Verification items for the finished model (mm, model axes). Face numbers are marked on the shaded views. A direction names the side the tool comes from. Give positions to 0.01 mm unless a question says otherwise; leave off trailing zeros. Loops run counter-clockwise (first coordinate to the right, second up) from the corner with the lowest first, then second, coordinate; pieces in that order, holes last. Notation, with made-up numbers: M -4.5,52.25 L 11.5,52.25 A26 cw 11.5,76.25 Z; hole C 69,-28.5 d10. An arc over 180 degrees is marked long. Use CSV: the item, a comma, the result in double quotes.
from build123d import *
from build123d.topology import SkipClean

# Parameters (mm, degrees)
BOSS_EXTRUDE1_DEPTH = 35
SKETCH2_W           = 14
SKETCH2_H           = 21
CUT_EXTRUDE1_DEPTH  = 35
BOSS_EXTRUDE2_DEPTH = 35
CUT_EXTRUDE2_DEPTH  = 58
FILLET1_R           = 5
CHAMFER2_SIZE       = 0.5
CHAMFER3_SIZE       = 0.5
CUT_EXTRUDE3_START  = -7
CUT_EXTRUDE3_DEPTH  = 3.2
CUT_EXTRUDE4_START  = -28
SKETCH4_3_R         = 2.5
CUT_EXTRUDE4_DEPTH  = 3.2


with BuildPart() as part:
    # Sketch1 → Boss-Extrude1 (new body)
    with BuildSketch(Plane.XY):
        with BuildLine():
            ThreePointArc((32.5, -4.75), (27.75, 0), (32.5, 4.75))
            Line((32.5, 4.75), (-32.5, 4.75))
            ThreePointArc((-32.5, 4.75), (-29.141242789, 3.358757211), (-27.75, 0))
            ThreePointArc((-27.75, 0), (-29.141242789, -3.358757211), (-32.5, -4.75))
            Line((-32.5, -4.75), (32.5, -4.75))
        make_face()
        with BuildLine():
            ThreePointArc((-27.75, 0), (-29.141242789, 3.358757211), (-32.5, 4.75))
            Line((-32.5, 4.75), (-32.5, 2))
            ThreePointArc((-32.5, 2), (-31.085786438, 1.414213562), (-30.5, 0))
            ThreePointArc((-30.5, 0), (-31.085786438, -1.414213562), (-32.5, -2))
            Line((-32.5, -2), (-32.5, -4.75))
            ThreePointArc((-32.5, -4.75), (-29.141242789, -3.358757211), (-27.75, 0))
        make_face()
        with BuildLine():
            Line((-32.5, 2), (-32.5, 4.75))
            ThreePointArc((-32.5, 4.75), (-35.858757211, 3.358757211), (-37.25, 0))
            ThreePointArc((-37.25, 0), (-35.858757211, -3.358757211), (-32.5, -4.75))
            Line((-32.5, -4.75), (-32.5, -2))
            ThreePointArc((-32.5, -2), (-34.5, 0), (-32.5, 2))
        make_face()
        with BuildLine():
            ThreePointArc((32.5, -4.75), (35.858757211, -3.358757211), (37.25, 0))
            ThreePointArc((37.25, 0), (35.858757211, 3.358757211), (32.5, 4.75))
            Line((32.5, 4.75), (32.5, 2))
            ThreePointArc((32.5, 2), (33.914213562, 1.414213562), (34.5, 0))
            ThreePointArc((34.5, 0), (33.914213562, -1.414213562), (32.5, -2))
            Line((32.5, -2), (32.5, -4.75))
        make_face()
        with BuildLine():
            Line((32.5, 2), (32.5, 4.75))
            ThreePointArc((32.5, 4.75), (27.75, 0), (32.5, -4.75))
            Line((32.5, -4.75), (32.5, -2))
            ThreePointArc((32.5, -2), (30.5, 0), (32.5, 2))
        make_face()
        with BuildLine():
            ThreePointArc((-37.25, 0), (-35.858757211, 3.358757211), (-32.5, 4.75))
            Line((-32.5, 4.75), (-34.942476014, 4.75))
            Line((-34.942476014, 4.75), (-37.25, 2))
            Line((-37.25, 2), (-37.25, 0))
        make_face()
        with BuildLine():
            Line((-34.942476014, -4.75), (-32.5, -4.75))
            ThreePointArc((-32.5, -4.75), (-35.858757211, -3.358757211), (-37.25, 0))
            Line((-37.25, 0), (-37.25, -2))
            Line((-37.25, -2), (-34.942476014, -4.75))
        make_face()
        with BuildLine():
            Line((37.25, 0), (37.25, 2))
            Line((37.25, 2), (34.942476014, 4.75))
            Line((34.942476014, 4.75), (32.5, 4.75))
            ThreePointArc((32.5, 4.75), (35.858757211, 3.358757211), (37.25, 0))
        make_face()
        with BuildLine():
            Line((37.25, -2), (37.25, 0))
            ThreePointArc((37.25, 0), (35.858757211, -3.358757211), (32.5, -4.75))
            Line((32.5, -4.75), (34.942476014, -4.75))
            Line((34.942476014, -4.75), (37.25, -2))
        make_face()
    extrude(amount=BOSS_EXTRUDE1_DEPTH)

    # Sketch2 → Cut-Extrude1 (cut)
    with BuildSketch(Plane(origin=(0, 4.75, 0), x_dir=(1, 0, 0), z_dir=(0, 1, 0))):
        with Locations((30.25, -17.5)):
            Rectangle(SKETCH2_W, SKETCH2_H)
        with Locations((-30.25, -17.5)):
            Rectangle(SKETCH2_W, SKETCH2_H)
    extrude(amount=-CUT_EXTRUDE1_DEPTH, mode=Mode.SUBTRACT)

    # Sketch3 → Boss-Extrude2 (add)
    with BuildSketch(Plane(origin=(0, 0, 0), x_dir=(-1, 0, 0), z_dir=(0, 0, -1))):
        with BuildLine():
            ThreePointArc((-5, 8.75), (-8.16227766, 7.622983346), (-9.898979486, 4.75))
            Line((-9.898979486, 4.75), (-5.830662386, 4.75))
            ThreePointArc((-5.830662386, 4.75), (-5, 5.05), (-4.169337614, 4.75))
            Line((-4.169337614, 4.75), (4.169337614, 4.75))
            ThreePointArc((4.169337614, 4.75), (5, 5.05), (5.830662386, 4.75))
            Line((5.830662386, 4.75), (9.898979486, 4.75))
            ThreePointArc((9.898979486, 4.75), (8.16227766, 7.622983346), (5, 8.75))
            Line((5, 8.75), (-5, 8.75))
        make_face()
    extrude(amount=-BOSS_EXTRUDE2_DEPTH)

    # Sketch3<2> → Cut-Extrude2 (cut)
    with SkipClean():  # the faces are left unmerged after this step: merging them gives an invalid solid
        with BuildSketch(Plane(origin=(0, 0, 0), x_dir=(-1, 0, 0), z_dir=(0, 0, -1))):
            with BuildLine():
                Line((0.830662386, 4.75), (-0.830662386, 4.75))
                ThreePointArc((-0.830662386, 4.75), (-0.552330923, 2.573169277), (1.3, 3.75))
                ThreePointArc((1.3, 3.75), (1.176830723, 4.302330923), (0.830662386, 4.75))
            make_face()
            with BuildLine():
                ThreePointArc((0.830662386, 4.75), (0, 5.05), (-0.830662386, 4.75))
                Line((-0.830662386, 4.75), (0.830662386, 4.75))
            make_face()
            with BuildLine():
                Line((-4.169337614, 4.75), (-5.830662386, 4.75))
                ThreePointArc((-5.830662386, 4.75), (-5.552330923, 2.573169277), (-3.7, 3.75))
                ThreePointArc((-3.7, 3.75), (-3.823169277, 4.302330923), (-4.169337614, 4.75))
            make_face()
            with BuildLine():
                ThreePointArc((-4.169337614, 4.75), (-5, 5.05), (-5.830662386, 4.75))
                Line((-5.830662386, 4.75), (-4.169337614, 4.75))
            make_face()
            with BuildLine():
                Line((4.169337614, 4.75), (5.830662386, 4.75))
                ThreePointArc((5.830662386, 4.75), (5, 5.05), (4.169337614, 4.75))
            make_face()
            with BuildLine():
                ThreePointArc((6.3, 3.75), (6.176830723, 4.302330923), (5.830662386, 4.75))
                Line((5.830662386, 4.75), (4.169337614, 4.75))
                ThreePointArc((4.169337614, 4.75), (4.447669077, 2.573169277), (6.3, 3.75))
            make_face()
        extrude(amount=-CUT_EXTRUDE2_DEPTH, mode=Mode.SUBTRACT)

    # Fillet1
    fillet1_edges = [part.edges().sort_by_distance(p)[0] for p in [
        (-9.898979486, 4.75, 17.5),
        (9.898979486, 4.75, 17.5),
    ]]
    fillet(fillet1_edges, radius=FILLET1_R)

    # Chamfer2
    chamfer2_edges = [part.edges().sort_by_distance(p)[0] for p in [
        (-6.176830723, 4.302330923, 0),
        (3.823169277, 4.302330923, 0),
        (7.236067977, 8.222135955, 35),
        (0, 8.75, 0),
        (7.236067977, 8.222135955, 0),
        (-4.447669077, 2.573169277, 35),
        (5.552330923, 2.573169277, 35),
        (0, 8.75, 35),
        (-23.971238007, 4.75, 35),
        (-32.5, -2, 0),
        (36.096238007, 3.375, 0),
        (37.25, 0, 0),
        (1.3, 3.75, 35),
        (1.3, 3.75, 0),
        (36.096238007, -3.375, 0),
        (0, -4.75, 0),
        (23.971238007, 4.75, 35),
        (23.971238007, 4.75, 0),
        (-7.236067977, 8.222135955, 35),
        (-7.236067977, 8.222135955, 0),
        (10.763932023, 5.277864045, 0),
        (10.763932023, 5.277864045, 35),
        (-10.763932023, 5.277864045, 0),
        (-10.763932023, 5.277864045, 35),
        (-36.096238007, -3.375, 0),
        (-37.25, 0, 0),
        (-36.096238007, 3.375, 0),
        (-23.971238007, 4.75, 0),
        (32.5, -2, 0),
        (-36.096238007, 3.375, 35),
        (-37.25, 0, 35),
        (-36.096238007, -3.375, 35),
        (0, -4.75, 35),
        (-23.25, -4.75, 17.5),
        (36.096238007, -3.375, 35),
        (37.25, 0, 35),
        (36.096238007, 3.375, 35),
        (-32.5, -2, 35),
        (32.5, -2, 35),
        (-37.25, 0, 28),
        (-23.25, 0, 7),
        (-36.096238007, 3.375, 7),
        (-29.096238007, -4.75, 7),
        (-36.096238007, -3.375, 7),
        (-37.25, 0, 7),
        (-32.5, -2, 7),
        (-36.096238007, 3.375, 28),
        (-36.096238007, -3.375, 28),
        (-29.096238007, -4.75, 28),
        (-23.25, 0, 28),
        (-32.5, -2, 28),
        (-29.096238007, 4.75, 7),
        (-29.096238007, 4.75, 28),
        (-23.25, 4.75, 17.5),
    ]]
    chamfer(chamfer2_edges, length=CHAMFER2_SIZE)

    # Chamfer3
    chamfer3_edges = [part.edges().sort_by_distance(p)[0] for p in [
        (23.25, -4.75, 17.5),
        (23.25, 4.75, 17.5),
    ]]
    chamfer(chamfer3_edges, length=CHAMFER3_SIZE)

    # Sketch4 → Cut-Extrude3 (cut)
    with SkipClean():  # the faces are left unmerged after this step: merging them gives an invalid solid
        with BuildSketch(Plane(origin=(0, 0, 0), x_dir=(-1, 0, 0), z_dir=(0, 0, -1)).offset(CUT_EXTRUDE3_START)):
            Polygon((-28.9, -2.078460969), (-28.9, 2.078460969), (-32.5, 4.156921938), (-32.5, 4.75), (-41.441027027, 4.75), (-41.441027027, -4.75), (-32.5, -4.75), (-32.5, -4.156921938), align=None)
        extrude(amount=CUT_EXTRUDE3_DEPTH, mode=Mode.SUBTRACT)

    # Sketch4<3> → Cut-Extrude4 (cut)
    # profile 1 of 3: a face of its own
    with SkipClean():  # the faces are left unmerged after this step: merging them gives an invalid solid
        with BuildSketch(Plane(origin=(0, 0, 0), x_dir=(-1, 0, 0), z_dir=(0, 0, -1)).offset(CUT_EXTRUDE4_START)):
            Polygon((-28.9, -2.078460969), (-28.9, 2.078460969), (-32.5, 4.156921938), (-32.5, 4.25), (-34.709322185, 4.25), (-36.75, 1.818014883), (-36.75, -1.818014883), (-34.709322185, -4.25), (-32.5, -4.25), (-32.5, -4.156921938), align=None)
            with Locations((-32.5, 0)):
                Circle(SKETCH4_3_R, mode=Mode.SUBTRACT)
        # profile 2 of 3: a face of its own
        with BuildSketch(Plane(origin=(0, 0, 0), x_dir=(-1, 0, 0), z_dir=(0, 0, -1)).offset(CUT_EXTRUDE4_START)):
            with Locations((-32.5, 0)):
                Circle(SKETCH4_3_R)
        # profile 3 of 3: a face of its own
        with BuildSketch(Plane(origin=(0, 0, 0), x_dir=(-1, 0, 0), z_dir=(0, 0, -1)).offset(CUT_EXTRUDE4_START)):
            Polygon((-34.709322185, 4.25), (-32.5, 4.25), (-32.5, 4.75), (-41.441027027, 4.75), (-41.441027027, -4.75), (-32.5, -4.75), (-32.5, -4.25), (-34.709322185, -4.25), (-36.75, -1.818014883), (-36.75, 1.818014883), align=None)
        extrude(amount=-CUT_EXTRUDE4_DEPTH, mode=Mode.SUBTRACT)


solid = part.part
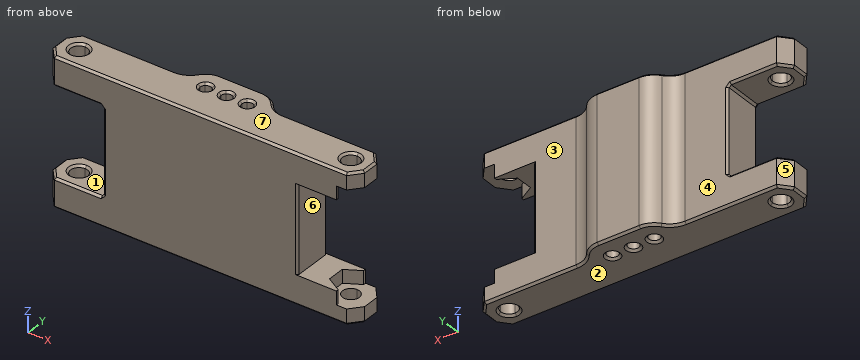
(1) Section check C-C on x = 18. Record the cut outline in (y, z).
Calculated:
outline,"M -4.75,0.5 L -4.25,0 L 4.25,0 L 4.75,0.5 L 4.75,34.5 L 4.25,35 L -4.25,35 L -4.75,34.5 Z"
(2) Mould release check, pull along Z, two halves, no side actions. Record for the marked faces 5, 6 and 7: released by +Z, released by -Z, zero draft, split by the parting line, or undercut.
Calculated:
face 5,"zero draft"
face 6,"undercut"
face 7,"released by +Z"
(3) Scan lines: L1, parallel to X at y = 3.75, z = 9; L2, parallel to Z at x = -30, y = -2.75; L3, parallel to X at y = 2.75, z = 15. Record each from-to range of solid material in increasing order. Write a range as from..to.
Calculated:
L1,"x = -23.25..-6.3, -3.7..-1.3, 1.3..3.7, 6.3..23.25"
L2,"z = 0..7, 28..35"
L3,"x = -23.25..-5.83, -4.17..-0.83, 0.83..4.17, 5.83..23.25"
(4) Section check A-A on x = -26. Record the cut outline in (y, z).
Calculated:
outline,"M -4.75,0.5 L -4.25,0 L 4.25,0 L 4.75,0.5 L 4.75,6.5 L 4.25,7 L -4.25,7 L -4.75,6.5 Z; M -4.75,28.5 L -4.25,28 L 4.25,28 L 4.75,28.5 L 4.75,34.5 L 4.25,35 L -4.25,35 L -4.75,34.5 Z"
(5) Section check B-B on z = 21. Record the cut outline in (x, y), plus the area to 3 significant figures.
Calculated:
outline,"M -23.25,-4.25 L -22.75,-4.75 L 22.75,-4.75 L 23.25,-4.25 L 23.25,4.25 L 22.75,4.75 L 13,4.75 A5 cw 9,6.75 A5 ccw 5,8.75 L -5,8.75 A5 ccw -9,6.75 A5 cw -13,4.75 L -22.75,4.75 L -23.25,4.25 Z; hole C -5,3.75 d2.6; hole C 0,3.75 d2.6; hole C 5,3.75 d2.6"
area,"497 mm²"
(6) Depth check by flat-ended pin: pin 1 Ø0.5 at (y, z) = (-4.5, 29) entering from +X; pin 2 Ø2 at (x, z) = (-17.5, 9.5) entering from +Y; pin 3 Ø7 at (y, z) = (1.5, 14) entering from -X. Enter the tip coordinate at first touch or a pass-through.
Calculated:
pin 1,"stops at x = 32.5"
pin 2,"stops at y = 4.75"
pin 3,"stops at x = -23.25"
(7) Section check D-D on x = 0. Record the cut outline in (y, z).
Calculated:
outline,"M -4.75,0.5 L -4.25,0 L 1.95,0 L 2.45,0.5 L 2.45,34.5 L 1.95,35 L -4.25,35 L -4.75,34.5 Z; M 5.05,0.5 L 5.55,0 L 8.25,0 L 8.75,0.5 L 8.75,34.5 L 8.25,35 L 5.55,35 L 5.05,34.5 Z"
(8) Tool access check on the marked faces 1, 2, 3 and 4. Record the directions out of +Z, -Z, +X, -X, +Y, -Y that give a thin tool (end or side, any length) a straight path to the whole face; none if there is none.
Calculated:
face 1,"-X, +Y, -Y"
face 2,"-Z, +X, -X, +Y, -Y"
face 3,"+Z, -Z, +X, +Y"
face 4,"+Z, -Z, -X, +Y"
